Could you check a few things on this model? Use its own coordinates, in mm. A direction names the side the tool comes from. Round coordinates to 2 decimals unless told otherwise and drop trailing zeros. Write each loop counter-clockwise with the first axis right and the second up, starting at its lowest first coordinate (ties: lowest second). Pieces come first, ordered by that corner, then holes. Notation, with made-up numbers: M 76.25,-1.5 L 133.25,-1.5 A26 ccw 133.25,18.5 Z; hole C -31,86.25 d2. An arc over 180 degrees is marked long. One line per item, written item: value. Start each with the question number.
(1) I want a section at A-A on z = 22. Please give me the cut outline in (x, y), and give its area (3 significant figures).
(2) If I drill on L1, parallel to Z at x = -82, y = 16; L2, parallel to X at y = 12.25, z = 51; L3, parallel to Z at x = -22, y = 2.5, over which ranges is the centre line in solid material (lowest first)?
(3) Which directions (+Z, -Z, +X, -X, +Y, -Y) give clear straight access to the entire face, cutting with the end or side of a thin tool? Please do faces 1 (the face through (-60.354, 1, -7)), 2 (the face through (-97, 14.5, 4)), 3 (the face through (-95.48, 10.12, -6.75)), 4 (the face through (-50, 10, 55.32)), 5 (the face through (-97, 0, 14)).
(4) I want a section at D-D on y = 18.5. Please give me the cut outline in (x, z).
(5) I want a section at C-C on x = -54.5. Please give me the cut outline in (y, z).
(6) I want a section at B-B on y = 11. Please give me the cut outline in (x, z).
(7) I'm going to push flat-ended pins straight in: pin 1 Ø2 at (y, z) = (4, 26) entering from -X; pin 2 Ø1.6 at (y, z) = (0.5, -7) entering from -X; pin 3 Ø0.6 at (x, z) = (-96.5, 25.5) entering from -Y. Where does each tip first touch, or does it pass through?
(8) Thinking about a two-plate mould opening in X: for faces 6 (the face through (-51, 10, 57.32)), 7 (the face through (-16.904, 2, -7)), 8 (the face through (-68.354, 1, -7)), 9 (the face through (-3.154, 10, 25)), which applies, released by +X, released by -X, zero draft, split by the parting line, or undercut?
```python
from build123d import *

# Parameters (mm, degrees)
BOSS_EXTRUDE1_DEPTH = 20.53
CUT_EXTRUDE1_REACH  = 112.841
SKETCH2_W           = 17
SKETCH2_H           = 14.5
SKETCH2_W_2         = 14.2
SKETCH2_H_2         = 16
CUT_EXTRUDE2_REACH  = 121.062
SKETCH3_W           = 9
SKETCH3_H           = 3.16
SKETCH3_W_2         = 16
SKETCH3_H_2         = 6.6


with BuildPart() as part:
    # Sketch1 → Boss-Extrude1 (new body)
    with BuildSketch(Plane(origin=(0, 0, 0), x_dir=(1, 0, 0), z_dir=(0, 1, 0))):
        with BuildLine():
            Line((-97.654422032, 2.625826009), (-97.654422032, -52.319988394))
            ThreePointArc((-97.654422032, -52.319988394), (-96.189955938, -55.8555223), (-92.654422032, -57.319988394))
            Line((-92.654422032, -57.319988394), (-8.154422032, -57.319988394))
            ThreePointArc((-8.154422032, -57.319988394), (-4.618888126, -55.8555223), (-3.154422032, -52.319988394))
            Line((-3.154422032, -52.319988394), (-3.154422032, 2.625826009))
            ThreePointArc((-3.154422032, 2.625826009), (-4.618888126, 6.161359915), (-8.154422032, 7.625826009))
            Line((-8.154422032, 7.625826009), (-92.654422032, 7.625826009))
            ThreePointArc((-92.654422032, 7.625826009), (-96.189955938, 6.161359915), (-97.654422032, 2.625826009))
        make_face()
        with BuildLine():
            Line((-92.654422032, 5.625826009), (-8.154422032, 5.625826009))
            ThreePointArc((-8.154422032, 5.625826009), (-6.033101689, 4.747146353), (-5.154422032, 2.625826009))
            Line((-5.154422032, 2.625826009), (-5.154422032, -52.319988394))
            ThreePointArc((-5.154422032, -52.319988394), (-6.033101689, -54.441308738), (-8.154422032, -55.319988394))
            Line((-8.154422032, -55.319988394), (-92.654422032, -55.319988394))
            ThreePointArc((-92.654422032, -55.319988394), (-94.775742376, -54.441308738), (-95.654422032, -52.319988394))
            Line((-95.654422032, -52.319988394), (-95.654422032, 2.625826009))
            ThreePointArc((-95.654422032, 2.625826009), (-94.775742376, 4.747146353), (-92.654422032, 5.625826009))
        make_face(mode=Mode.SUBTRACT)
    extrude(amount=BOSS_EXTRUDE1_DEPTH)

    # Sketch2 → Cut-Extrude1 (cut, up to next)
    with BuildSketch(Plane(origin=(-97.654422032, 0, 3.154422032), x_dir=(0, 0, 1), z_dir=(-1, 0, 0)), mode=Mode.PRIVATE) as cut_extrude1_sk1:
        with Locations((0.619751959, 7.25)):
            Rectangle(SKETCH2_W, SKETCH2_H)
    cut_extrude1_tool1 = extrude(cut_extrude1_sk1.sketch, amount=-CUT_EXTRUDE1_REACH, mode=Mode.PRIVATE) & part.part
    # Sketch2 → Cut-Extrude1 (cut, up to next)
    with BuildSketch(Plane(origin=(-97.654422032, 0, 3.154422032), x_dir=(0, 0, 1), z_dir=(-1, 0, 0)), mode=Mode.PRIVATE) as cut_extrude1_sk2:
        with Locations((19.419751959, 8)):
            Rectangle(SKETCH2_W_2, SKETCH2_H_2)
    cut_extrude1_tool2 = extrude(cut_extrude1_sk2.sketch, amount=-CUT_EXTRUDE1_REACH, mode=Mode.PRIVATE) & part.part
    # Sketch2 → Cut-Extrude1 (cut, up to next)
    with BuildSketch(Plane(origin=(-97.654422032, 0, 3.154422032), x_dir=(0, 0, 1), z_dir=(-1, 0, 0)), mode=Mode.PRIVATE) as cut_extrude1_sk3:
        with Locations((37.469751959, 8)):
            Rectangle(SKETCH2_W_2, SKETCH2_H_2)
    cut_extrude1_tool3 = extrude(cut_extrude1_sk3.sketch, amount=-CUT_EXTRUDE1_REACH, mode=Mode.PRIVATE) & part.part
    add(cut_extrude1_tool1.solids().sort_by_distance((-97.654422, 7.25, 3.774174))[0], mode=Mode.SUBTRACT)
    add(cut_extrude1_tool2.solids().sort_by_distance((-97.654422, 8, 22.574174))[0], mode=Mode.SUBTRACT)
    add(cut_extrude1_tool3.solids().sort_by_distance((-97.654422, 8, 40.624174))[0], mode=Mode.SUBTRACT)

    # Sketch3 → Cut-Extrude2 (cut, up to next)
    with BuildSketch(Plane.XY.offset(-7.625826009), mode=Mode.PRIVATE) as cut_extrude2_sk1:
        with Locations((-21.404422032, 1.58)):
            Rectangle(SKETCH3_W, SKETCH3_H)
    cut_extrude2_tool1 = extrude(cut_extrude2_sk1.sketch, amount=CUT_EXTRUDE2_REACH, mode=Mode.PRIVATE) & part.part
    # Sketch3 → Cut-Extrude2 (cut, up to next)
    with BuildSketch(Plane.XY.offset(-7.625826009), mode=Mode.PRIVATE) as cut_extrude2_sk2:
        with Locations((-42.654422032, 3.3)):
            Rectangle(SKETCH3_W_2, SKETCH3_H_2)
    cut_extrude2_tool2 = extrude(cut_extrude2_sk2.sketch, amount=CUT_EXTRUDE2_REACH, mode=Mode.PRIVATE) & part.part
    # Sketch3 → Cut-Extrude2 (cut, up to next)
    with BuildSketch(Plane.XY.offset(-7.625826009), mode=Mode.PRIVATE) as cut_extrude2_sk3:
        with BuildLine():
            Line((-68.354422032, 0), (-60.354422032, 0))
            Line((-60.354422032, 0), (-60.354422032, 2.1))
            ThreePointArc((-60.354422032, 2.1), (-64.354422032, 6.1), (-68.354422032, 2.1))
            Line((-68.354422032, 2.1), (-68.354422032, 0))
        make_face()
    cut_extrude2_tool3 = extrude(cut_extrude2_sk3.sketch, amount=CUT_EXTRUDE2_REACH, mode=Mode.PRIVATE) & part.part
    add(cut_extrude2_tool1.solids().sort_by_distance((-21.404422, 1.58, -7.625826))[0], mode=Mode.SUBTRACT)
    add(cut_extrude2_tool2.solids().sort_by_distance((-42.654422, 3.3, -7.625826))[0], mode=Mode.SUBTRACT)
    add(cut_extrude2_tool3.solids().sort_by_distance((-64.354422, 2.696829, -7.625826))[0], mode=Mode.SUBTRACT)


solid = part.part
```
Found:
1. outline: M -97.65,16 L -95.65,16 L -95.65,20.53 L -97.65,20.53 Z; M -5.15,0 L -3.15,0 L -3.15,20.53 L -5.15,20.53 Z
1. area: 50.1 mm²
2. L1: z = -7.63 to -5.63, 55.32 to 57.32
2. L2: x = -97.65 to -95.65, -5.15 to -3.15
2. L3: z = 55.32 to 57.32
3. face 1: -Z, -Y
3. face 2: -X, -Y
3. face 3: -Z, -X, +Y, -Y
3. face 4: +Y, -Y
3. face 5: +Z, -Z, +X, -X, -Y
4. outline: M -97.65,-2.63 A5 ccw -92.65,-7.63 L -8.15,-7.63 A5 ccw -3.15,-2.63 L -3.15,52.32 A5 ccw -8.15,57.32 L -92.65,57.32 A5 ccw -97.65,52.32 Z; hole M -95.65,-2.63 A3 ccw -92.65,-5.63 L -8.15,-5.63 A3 ccw -5.15,-2.63 L -5.15,52.32 A3 ccw -8.15,55.32 L -92.65,55.32 A3 ccw -95.65,52.32 Z
5. outline: M 0,-7.63 L 20.53,-7.63 L 20.53,-5.63 L 0,-5.63 Z; M 0,55.32 L 20.53,55.32 L 20.53,57.32 L 0,57.32 Z
6. outline: M -97.65,12.27 L -95.65,12.27 L -95.65,15.47 L -97.65,15.47 Z; M -97.65,29.67 L -95.65,29.67 L -95.65,33.52 L -97.65,33.52 Z; M -97.65,47.72 L -95.65,47.72 L -95.65,52.32 A3 cw -92.65,55.32 L -8.15,55.32 A3 cw -5.15,52.32 L -5.15,-2.63 A3 cw -8.15,-5.63 L -92.65,-5.63 A3 cw -94.8,-4.73 L -97.19,-4.73 A5 ccw -92.65,-7.63 L -8.15,-7.63 A5 ccw -3.15,-2.63 L -3.15,52.32 A5 ccw -8.15,57.32 L -92.65,57.32 A5 ccw -97.65,52.32 Z
7. pin 1: stops at x = -5.15
7. pin 2: stops at x = -96.15
7. pin 3: stops at y = 16
8. face 6: zero draft
8. face 7: undercut
8. face 8: undercut
8. face 9: released by +X
